```python
from build123d import *

# Parameters (mm, degrees)
F0_W     = 5.1181
F0_H     = 5.1308
F1_DEPTH = 25.4


with BuildPart() as f1:
    # F0 (on Top) → F1 (new body)
    with BuildSketch(Plane.XY):
        Polygon((-18.632969, 30.72453), (6.960761, 5.1308), (12.078861, 10.2362), (-8.457507, 30.72161), align=None)
        Polygon((32.564271, 30.772569), (12.078861, 10.2362), (17.196961, 5.1308), (42.758878, 30.756304), align=None)
        Polygon((12.078861, 10.2362), (12.078861, 5.1308), (17.196961, 5.1308), align=None)
        Polygon((12.078861, 10.2362), (6.960761, 5.1308), (12.078861, 5.1308), align=None)
        Polygon((6.960761, 5.1308), (1.829961, 0), (6.960761, 0), align=None)
        with Locations((9.519811, 2.5654)):
            Rectangle(F0_W, F0_H)
        with Locations((14.637911, 2.5654)):
            Rectangle(F0_W, F0_H)
        Polygon((17.196961, 5.1308), (17.196961, 0), (22.327761, 0), align=None)
    extrude(amount=F1_DEPTH)


solid = f1.part
```
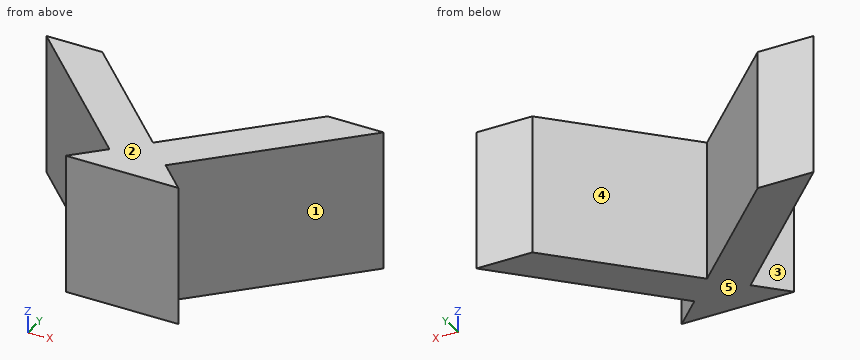
Build history of the part. All positions in model axes, mm. Face numbers are marked on the shaded views. A direction names the side the tool comes from. Round coordinates to 2 decimals unless told otherwise and drop trailing zeros. Loops run counter-clockwise (first coordinate to the right, second up) from the corner with the lowest first, then second, coordinate; pieces in that order, holes last.
Item 1: Saw through at A-A (y = 24.5). List the corners of the cut face in (x, z), then the cut area to 3 significant figures.
Item 2: Saw through at C-C (z = 11.75). List the corners of the cut face in (x, y), then the cut area to 3 significant figures.
Item 3: Which spindle directions (+Z, -Z, +X, -X, +Y, -Y) get a long thin tool onto all of the face, cutting with end or side? Do the marked faces 1, 2, 3, 4 and 5. Say none if no direction does.
Item 4: Pin check, flat tips, straight feed: P1, Ø6, axis at x = 7.5, z = 4, coming from the +Y side; P2, Ø1, axis at x = -3, z = 3.5, coming from the +Y side; P3, Ø1, axis at x = 1, z = 11.5, coming from the +Y side. Stop position of each tip, or through.
Item 5: Drill centre lines: line 1 along X through (y, z) = (17, 14.25); line 2 along X through (y, z) = (28.5, 10.75); line 3 along Y through (x, z) = (26.5, 5.75). Where is each one in solid material? Low to high.
Item 6: Saw through at B-B (x = 20). List the corners of the cut face in (y, z).
Item 7: Saw through at D-D (x = 1). List the corners of the cut face in (y, z), then the cut area to 3 significant figures.
Worked answers:
1. outline: (-12.41, 0) - (-2.22, 0) - (-2.22, 25.4) - (-12.41, 25.4) - close; (26.31, 0) - (36.52, 0) - (36.52, 25.4) - (26.31, 25.4) - close
1. area: 518 mm2
2. outline: (-18.63, 30.72) - (6.96, 5.13) - (1.83, 0) - (22.33, 0) - (17.2, 5.13) - (42.76, 30.76) - (32.56, 30.77) - (12.08, 10.24) - (-8.46, 30.72) - close
2. area: 576 mm2
3. face 1: +Z, -Z, +X
3. face 2: +Z, +X, -X, +Y, -Y
3. face 3: +Z, -Z, -X
3. face 4: +Z, -Z, +Y
3. face 5: -Z, +X, -X, +Y, -Y
4. P1: stops at y = 17.8
4. P2: stops at y = 25.78
4. P3: stops at y = 21.79
5. line 1: x = -4.91 to 5.3, 18.83 to 29.04
5. line 2: x = -16.41 to -6.23, 30.3 to 40.51
5. line 3: y = 14.46 to 24.69
6. outline: (0, 0) - (2.33, 0) - (2.33, 25.4) - (0, 25.4) - close; (7.94, 0) - (18.18, 0) - (18.18, 25.4) - (7.94, 25.4) - close
7. outline: (11.09, 0) - (21.29, 0) - (21.29, 25.4) - (11.09, 25.4) - close
7. area: 259 mm2
